Here's how the part is built. I have some questions about the finished solid (model axes, mm). Face numbers are marked on the shaded views. Round coordinates to 2 decimals unless told otherwise and drop trailing zeros. Write each loop counter-clockwise with the first axis right and the second up, starting at its lowest first coordinate (ties: lowest second). Pieces come first, ordered by that corner, then holes. Notation, with made-up numbers: (17.5, -17.5) -> (57.5, -17.5) arc R20 cw to (57.5, 18.5) -> close; hole circle Ø5 at (-10, -40). An arc over 180 degrees is marked (long way). Answer in a Markdown table with one row per item.
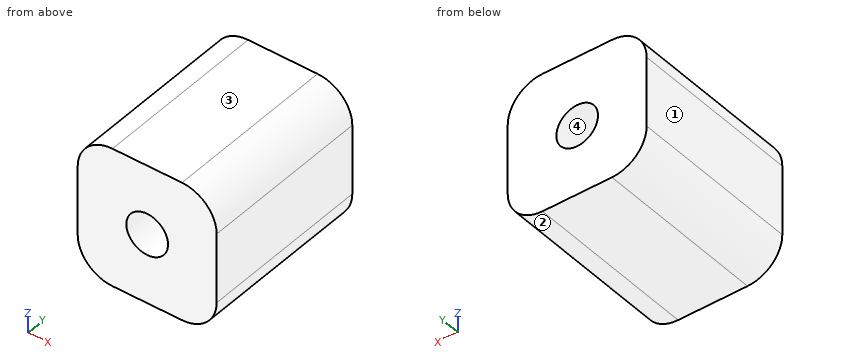
Autodesk Inventor part; units mm, degrees
ref_plane "YZ Plane" through (0, 0, 0) normal (1, 0, 0) x (0, 1, 0)
ref_plane "XZ Plane" through (0, 0, 0) normal (0, 1, 0) x (-1, 0, 0)
ref_plane "XY Plane" through (0, 0, 0) normal (0, 0, 1) x (1, 0, 0)
sketch "Sketch1" plane through (0, 0, 0) normal (0, 1, 0) x (-1, 0, 0)
  line L0 (0, 0) -> (20, 0)
  line L1 (20, 0) -> (20, -20)
  line L2 (20, -20) -> (0, -20)
  line L3 (0, -20) -> (0, 0)
  dimension "d0" = 20
  dimension "d1" = 20
extrude "Extrusion1" add sketch "Sketch1" along normal blind 25
sketch "Sketch2" plane through (0, 25, 0) normal (0, 1, 0) x (1, 0, 0)
  circle A0 centre (-10, 10) radius 3
  line L0 (0, 20) -> (-20, 20)
  line L1 (-20, 20) -> (-20, 0)
  point P0 (0, 0)
  dimension "d4" = 6
  dimension "d5" = 10
  dimension "d6" = 10
extrude "Extrusion2" cut sketch "Sketch2" against normal through all
fillet "Fillet1" radius 5 4 edges at (-20, 12.5, -20) (0, 12.5, 0) (0, 12.5, -20) (-20, 12.5, 0)
properties part number "SpacerBlock_25mm"
1) I need wall thicknesses on line 1 (X direction, y = 14.5, z = -10); line 2 (X direction, y = 20.75, z = -12.5). Which ranges of each line are inside material? Lowest first, please. Write a range as [from, to].
Response:
| item | result |
|---|---|
| line 1 | x = [-20, -13], [-7, 0] |
| line 2 | x = [-20, -11.66], [-8.34, 0] |
2) I want a section at C-C, the plane x = -10. List the corners of the cut face in (y, z) for me.
Response:
| item | result |
|---|---|
| outline | (0, -20) -> (25, -20) -> (25, -13) -> (0, -13) -> close; (0, -7) -> (25, -7) -> (25, 0) -> (0, 0) -> close |
3) For pin 1 (5 mm diameter, centred on y = 9, z = -18, fed in from -X), with a flat end and sliding along its axis, tell me the tip position at first contact or that it passes through.
Response:
| item | result |
|---|---|
| pin 1 | stops at x = -19.97 |
4) I want a section at A-A, the plane z = -10. List the corners of the cut face in (x, y) for me.
Response:
| item | result |
|---|---|
| outline | (-20, 0) -> (-13, 0) -> (-13, 25) -> (-20, 25) -> close; (-7, 0) -> (0, 0) -> (0, 25) -> (-7, 25) -> close |
5) I want a section at D-D, the plane z = -16.5. List the corners of the cut face in (x, y) for me.
Response:
| item | result |
|---|---|
| outline | (-19.77, 0) -> (-0.23, 0) -> (-0.23, 25) -> (-19.77, 25) -> close |
6) I want a section at B-B, the plane y = 13.25. List the corners of the cut face in (x, z) for me.
Response:
| item | result |
|---|---|
| outline | (-20, -15) arc R5 ccw to (-15, -20) -> (-5, -20) arc R5 ccw to (0, -15) -> (0, -5) arc R5 ccw to (-5, 0) -> (-15, 0) arc R5 ccw to (-20, -5) -> close; hole circle Ø6 at (-10, -10) |
7) We'd pull the mould along Z, two halves only. Please class the marked faces 1, 2, 3 and 4: +Z half, -Z half, draft (parallel to the pull), parting line (faces both ways), or undercut.
Response:
| item | result |
|---|---|
| face 1 | draft |
| face 2 | -Z half |
| face 3 | +Z half |
| face 4 | undercut |
